Geometry check sheet. Reference: the model listing, model coordinates, mm. A direction names the side the tool comes from. Give positions to 0.01 mm unless a question says otherwise; leave off trailing zeros. Write each loop counter-clockwise with the first axis right and the second up, starting at its lowest first coordinate (ties: lowest second). Pieces come first, ordered by that corner, then holes. Notation, with made-up numbers: (53, 35.25) -> (99, 35.25) arc R22 ccw to (99, 74.25) -> close; hole circle Ø3 at (-38, 11.5). An arc over 180 degrees is marked (long way). Write item = value, one per line. Start each with the question number.
1. Cross-section at B-B, the plane y = -165. Record the cut outline in (x, z).
2. Set-up check for faces 1 (the flat face through (-11.112, 4, 0)), 2 (the flat face through (-11.3, 254, -0.1)): record each of +Z, -Z, +X, -X, +Y, -Y from which the full face is reachable in a straight line by a thin tool's end or side.
3. Cross-section at A-A, the plane z = -7. Record the cut outline in (x, y).
4. Thickness scan on line 1 along Y through (x, z) = (0, -12.15) (3 decimals); line 2 along X through (y, z) = (-228.6, -11.95); line 3 along Z through (x, y) = (-0.25, -61.5). Record the ranges inside material, lowest first.
5. Mould release check, pull along Z, two halves, no side actions. Record for faces 3 (the flat face through (0, 4, 12.7)), 4 (the flat face through (0, 4, -12.7)), 5 (the flat face through (11.112, 4, 0)): pulls with the +Z half, pulls with the -Z half, needs draft (parallel to the pull), parting line crosses it, or undercut.
6. Cross-section at C-C, the plane x = 6.75. Record the cut outline in (y, z), plus the area to 3 significant figures.
7. Depth check by flat-ended pin: P1, Ø4, axis at x = 0, y = 228.6, coming from the -Z side. Enter the tip coordinate at first touch or a pass-through.
```python
from build123d import *

# Parameters (mm, degrees)
SKETCH1_W                        = 25.4
SKETCH1_H                        = 25.4
SKETCH1_W_2                      = 22.225
SKETCH1_H_2                      = 22.225
BOSS_EXTRUDE1_DEPTH              = 254
F_10_0_1935_DIAMETER_HOLE1_D     = 4.9149
F_10_0_1935_DIAMETER_HOLE1_DEPTH = 50.8
F_10_0_1935_DIAMETER_HOLE1_TIP   = 1.476584928
SKETCH6_R                        = 1.905
CUT_EXTRUDE1_DEPTH               = 256.582569828


with BuildPart() as part:
    # Sketch1 → Boss-Extrude1 (new, symmetric)
    with BuildSketch(Plane(origin=(0, 0, 0), x_dir=(1, 0, 0), z_dir=(0, 1, 0))):
        Rectangle(SKETCH1_W, SKETCH1_H)
        Rectangle(SKETCH1_W_2, SKETCH1_H_2, mode=Mode.SUBTRACT)
    extrude(amount=BOSS_EXTRUDE1_DEPTH, both=True)

    # #10 (0.1935) Diameter Hole1
    with Locations(Plane(origin=(0, 0, -12.7), x_dir=(-1, 0, 0), z_dir=(0, 0, -1))):
        with Locations((0, 228.6), (0, -228.6)):
            Hole(F_10_0_1935_DIAMETER_HOLE1_D / 2, depth=F_10_0_1935_DIAMETER_HOLE1_DEPTH)
            with Locations((0, 0, -(F_10_0_1935_DIAMETER_HOLE1_DEPTH + F_10_0_1935_DIAMETER_HOLE1_TIP / 2))):  # 118° drill point
                Cone(0, F_10_0_1935_DIAMETER_HOLE1_D / 2, F_10_0_1935_DIAMETER_HOLE1_TIP, mode=Mode.SUBTRACT)

    # Sketch6 → Cut-Extrude1 (cut, through all)
    with BuildSketch(Plane.XY.offset(12.7)):
        with Locations((0, -69.85)):
            Circle(SKETCH6_R)
        Circle(SKETCH6_R)
        with Locations((0, 69.85)):
            Circle(SKETCH6_R)
    extrude(amount=-CUT_EXTRUDE1_DEPTH, mode=Mode.SUBTRACT)


solid = part.part
```
Answers:
q1.outline = (-12.7, -12.7) -> (12.7, -12.7) -> (12.7, 12.7) -> (-12.7, 12.7) -> close; hole (-11.11, -11.11) -> (11.11, -11.11) -> (11.11, 11.11) -> (-11.11, 11.11) -> close
q2.face_1 = +Y, -Y
q2.face_2 = +Z, -Z, +X, -X, +Y
q3.outline = (-12.7, -254) -> (-11.11, -254) -> (-11.11, 254) -> (-12.7, 254) -> close; (11.11, -254) -> (12.7, -254) -> (12.7, 254) -> (11.11, 254) -> close
q4.line_1 = -254 to -231.057, -226.143 to -71.755, -67.945 to -1.905, 1.905 to 67.945, 71.755 to 226.143, 231.057 to 254
q4.line_2 = -12.7 to -2.46, 2.46 to 12.7
q4.line_3 = -12.7 to -11.11, 11.11 to 12.7
q5.face_3 = pulls with the +Z half
q5.face_4 = pulls with the -Z half
q5.face_5 = undercut
q6.outline = (-254, -12.7) -> (254, -12.7) -> (254, -11.11) -> (-254, -11.11) -> close; (-254, 11.11) -> (254, 11.11) -> (254, 12.7) -> (-254, 12.7) -> close
q6.area = 1,610 mm^2
q7.P1 = through
